from build123d import *
from build123d.topology import SkipClean

# Parameters (mm, degrees)
CIRPATTERN1_COUNT            = 8
SKETCH55_R                   = 2.175
CUT_EXTRUDE37_DEPTH          = 17.800398408
SCHIZZO1_R                   = 3.175
SCHIZZO1_R_2                 = 2.175
ESTRUSIONE_ESTRUSIONE1_DEPTH = 10
ESTRUSIONE_ESTRUSIONE2_START = 40
ESTRUSIONE_ESTRUSIONE2_DEPTH = 40
RACCORDO1_R                  = 8
SCHIZZO3_R                   = 3.175
TAGLIO_ESTRUSIONE1_DEPTH     = 14


with BuildPart() as part:
    # Sketch18 → Revolve1 (revolve)
    with BuildSketch(Plane(origin=(0, 0, 0), x_dir=(1, 0, 0), z_dir=(0, 1, 0)), mode=Mode.PRIVATE) as revolve1_sk:
        with BuildLine():
            Line((0, 88), (0, 80))
            ThreePointArc((0, 80), (-49.497474683, 59.497474683), (-70, 10))
            Line((-70, 10), (-70, -10))
            Line((-70, -10), (-72, -10))
            Line((-72, -10), (-72, 0))
            Line((-72, 0), (-73, 0))
            Line((-73, 0), (-73, 10))
            Line((-73, 10), (-73, 70.199601592))
            Line((-73, 70.199601592), (-41.29174213, 70.199601592))
            ThreePointArc((-41.29174213, 70.199601592), (-33.410035677, 74.90585117), (-25, 78.585712798))
            Line((-25, 78.585712798), (-25, 88))
            Line((-25, 88), (0, 88))
        make_face()
    revolve(revolve1_sk.sketch.rotate(Axis((0, 0, 0), (0, 0, -1)), 180), axis=Axis((0, 0, 0), (0, 0, -1)))

    # Sketch23 → Ø4.0 (4) Diameter Hole1 (revolve, cut)
    with BuildSketch(Plane(origin=(0, 73, -60.199601592), x_dir=(0, 0, 1), z_dir=(1, 0, 0))):
        Polygon((0, 0), (0, 16.3), (2, 14.3), (2, 0), align=None)
    f_4_0_4_diameter_hole1 = revolve(axis=Axis((0, 79.35, -60.199601592), (0, -1, 0)), mode=Mode.SUBTRACT)

    # CirPattern1: Ø4.0 (4) Diameter Hole1 ×8 about axis
    cirpattern1_axis = Axis((0, 0, 0), (0, 0, -1))
    for i in range(1, CIRPATTERN1_COUNT):
        add(f_4_0_4_diameter_hole1.rotate(cirpattern1_axis, i * 360 / CIRPATTERN1_COUNT), mode=Mode.SUBTRACT)

    # Sketch55 → Cut-Extrude37 (cut)
    with BuildSketch(Plane(origin=(0, 0, -70.199601592), x_dir=(-1, 0, 0), z_dir=(0, 0, -1))):
        with Locations(Location((0, 0, 0), (0, 0, 180))):
            Circle(SKETCH55_R)
    extrude(amount=CUT_EXTRUDE37_DEPTH, mode=Mode.SUBTRACT)

    # Fillet8: read off the stored shape, not the designer's step
    # Fillet8 outline → Fillet8 (revolve, cut)
    with BuildSketch(Plane.XZ):
        with BuildLine():
            ThreePointArc((2.175, -82.816340027), (2.979776356, -80.771592329), (4.962328767, -79.823887698))
            Line((4.962328767, -79.823887698), (2.175, -79.823887698))
            Line((2.175, -79.823887698), (2.175, -82.816340027))
        make_face()
    revolve(axis=Axis((0, 0, 0), (0, 0, 1)), mode=Mode.SUBTRACT)

    # Schizzo1 → Estrusione-Estrusione1 (add)
    with BuildSketch(Plane(origin=(0, 0, -88), x_dir=(-1, 0, 0), z_dir=(0, 0, -1))):
        with Locations(Location((0, 0, 0), (0, 0, 180))):
            Circle(SCHIZZO1_R)
        with Locations(Location((0, 0, 0), (0, 0, 180))):
            Circle(SCHIZZO1_R_2, mode=Mode.SUBTRACT)
    extrude(amount=ESTRUSIONE_ESTRUSIONE1_DEPTH)

    # Schizzo2 → Estrusione-Estrusione2 (add)
    with BuildSketch(Plane(origin=(0, 0, -70.199601592), x_dir=(-1, 0, 0), z_dir=(0, 0, -1)).offset(ESTRUSIONE_ESTRUSIONE2_START)):
        with BuildLine():
            ThreePointArc((3.496742934, 72.916203884), (-2.871629137, 72.943496942), (-9.218146375, 72.415645943))
            Line((-9.218146375, 72.415645943), (-8.586766487, 67.455670194))
            ThreePointArc((-8.586766487, 67.455670194), (-2.674942209, 67.947367014), (3.257239993, 67.921943344))
            Line((3.257239993, 67.921943344), (3.496742934, 72.916203884))
        make_face()
        with BuildLine():
            Line((-8.586766487, 67.455670194), (-9.218146375, 72.415645943))
            ThreePointArc((-9.218146375, 72.415645943), (-15.494507954, 71.336668154), (-21.652946971, 69.714775245))
            Line((-21.652946971, 69.714775245), (-20.169868412, 64.939790639))
            ThreePointArc((-20.169868412, 64.939790639), (-14.433240286, 66.450594992), (-8.586766487, 67.455670194))
        make_face()
    extrude(amount=-ESTRUSIONE_ESTRUSIONE2_DEPTH)

    # Raccordo1
    raccordo1_edges = [part.edges().sort_by_distance(p)[0] for p in [
        (20.911407692, 67.327282942, -110.199601592),
        (-3.376991464, 70.419073614, -110.199601592),
    ]]
    fillet(raccordo1_edges, radius=RACCORDO1_R)

    # Schizzo3 → Taglio-Estrusione1 (cut)
    with SkipClean():  # the faces are left unmerged after this step: merging them gives an invalid solid
        with BuildSketch(Plane(origin=(13.072496691, 62.257996798, 0), x_dir=(0.978658816176937, -0.20549190134688128, 0), z_dir=(0.2054919013468813, 0.9786588161769371, 0))):
            with Locations((-6.110316561, 97.844831396)):
                Circle(SCHIZZO3_R)
        extrude(amount=TAGLIO_ESTRUSIONE1_DEPTH, mode=Mode.SUBTRACT)


solid = part.part
Can you work these out from the model? Positions are in its coordinate system, mm. A direction names the side the tool comes from. Coordinates: 2 decimals unless noted, no trailing zeros. Write each loop counter-clockwise with the first axis right and the second up, starting at its lowest first coordinate (ties: lowest second). Pieces come first, ordered by that corner, then holes. Notation, with made-up numbers: (50, 42.25) -> (86, 42.25) arc R4 cw to (86, 48.25) -> close; hole circle Ø1 at (-25.75, 5.5). An arc over 180 degrees is marked (long way). Write each question's results on one line, items separated by ' | '. Start each with the question number.
Q1. I'm going to push flat-ended pins straight in: pin 1 (4.5 mm diameter, centred on x = 0, z = -60.2, fed in from +Y); pin 2 (2 mm diameter, centred on y = 13, z = -56, fed in from +X); pin 3 (1 mm diameter, centred on x = 51.5, y = 37.5, fed in from -Z); pin 4 (2 mm diameter, centred on y = 37, z = -22.5, fed in from -X). Where does each tip first touch, or does it pass through?
Q2. If I drill on probe 1 along Y at (x, z) = (57.5, -32.5) (3 decimals); probe 2 along Y at (x, z) = (-2.5, -67); probe 3 along Z at (x, y) = (58, -0.5), over which ranges is the centre line in solid material (lowest first)?
Q3. Imagine slicing it at C-C (x = -38). Write out the boundary of the cut face in (y, z).
Q4. We'd pull the mould along Z, two halves only. Please class faces 5 (the face through (-3.375, 70.384, -86.424)), 6 (the face through (-57.27, -0.385, -60.619)), 7 (the face through (0.088, -65.95, -62.198)), 8 (the face through (-54, 48, 0)): +Z half, -Z half, draft (parallel to the pull), parting line (faces both ways), or undercut.
Q5. Imagine slicing it at D-D (y = 23). Write out the boundary of the cut face in (x, z).
Q6. Imagine slicing it at A-A (z = -91). Write out the boundary of the cut face in (x, y) (3 decimals), then the cut area to 3 significant figures.
Q7. On a 3-axis mill with a long thin cutter (end or side, diameter ignored), from which of +Z, -Z, +X, -X, +Y, -Y can I reach the whole of each face in a straight line? I mean faces 1 (the face through (-15.175, 68.335, 0.14)), 2 (the face through (20.92, 67.36, -86.42)), 3 (the face through (-65.95, -0.088, -62.198)), 4 (the face through (31, 31, -70.2)). Say none if no direction works.
Q8. Imagine slicing it at B-B (y = -63). Write out the boundary of the cut face in (x, z).
Taken from the geometry:
1) pin 1: stops at y = 73 | pin 2: stops at x = 72.01 | pin 3: stops at z = -70.2 | pin 4: stops at x = -63.51
2) probe 1: y = -44.975 to -32.977, 32.977 to 44.975 | probe 2: y = -72.96 to -40.56, 40.56 to 72.96 | probe 3: z = -70.2 to -61.4, -59 to -49.19
3) outline: (-62.33, -70.2) -> (-16.16, -70.2) arc R62.33 ccw to (16.16, -70.2) -> (62.33, -70.2) -> (62.33, 0) -> (61.16, 0) -> (61.16, 10) -> (58.79, 10) -> (58.79, -10) arc R58.79 cw to (-58.79, -10) -> (-58.79, 10) -> (-61.16, 10) -> (-61.16, 0) -> (-62.33, 0) -> close
4) face 5: draft | face 6: undercut | face 7: undercut | face 8: +Z half
5) outline: (-69.28, -70.2) -> (-34.29, -70.2) arc R69.28 ccw to (-9.8, -78.59) -> (-9.8, -88) -> (9.8, -88) -> (9.8, -78.59) arc R69.28 ccw to (34.29, -70.2) -> (69.28, -70.2) -> (69.28, 0) -> (68.23, 0) -> (68.23, 10) -> (66.11, 10) -> (66.11, -10) arc R66.11 cw to (-66.11, -10) -> (-66.11, 10) -> (-68.23, 10) -> (-68.23, 0) -> (-69.28, 0) -> close
6) outline: (-3.497, 72.916) -> (-3.257, 67.922) arc R68 cw to (20.17, 64.94) -> (21.653, 69.715) arc R73 ccw to start; circle Ø6.35 at (0, 0); hole circle Ø4.35 at (0, 0) | area: 140 mm^2
7) face 1: +Z | face 2: -Z, +X | face 3: -X | face 4: -Z
8) outline: (-36.88, -70.2) -> (36.88, -70.2) -> (36.88, 0) -> (34.86, 0) -> (34.86, 10) -> (30.51, 10) -> (30.51, -10) arc R30.51 cw to (-30.51, -10) -> (-30.51, 10) -> (-34.86, 10) -> (-34.86, 0) -> (-36.88, 0) -> close; hole circle Ø4 at (0, -60.2)
